Source: CAD feature listing. Evaluate the final solid. Frame: model axes, mm. A direction names the side the tool comes from. Coordinates: 2 decimals unless noted, no trailing zeros. Loops run counter-clockwise (first coordinate to the right, second up) from the corner with the lowest first, then second, coordinate; pieces in that order, holes last.
Item 1: Section query C-C, the plane x = 50. Return the cut outline in (y, z), then the cut area to 3 significant figures.
Item 2: Pull-direction query (Y, two-part tool) for faces 3 (the cylindrical face through (8.73, 42.03, 1.52)), 4 (the flat face through (30, 53, 1)), 5 (the flat face through (0, 26, 1)), 6 (the cylindrical face through (59, 2, 2)); classes: +Y half, -Y half, draft (parallel to the pull), parting line (faces both ways), or undercut.
Item 3: Reachability of faces 1 (the flat face through (60, 26, 1)), 2 (the flat face through (40, 24, 2)) from +Z, -Z, +X, -X, +Y, -Y: full face, straight path, thin tool, end or side. Return the list, or none.
Item 4: Section query D-D, the plane z = 0.65. Return the cut outline in (x, y).
Item 5: Section query B-B, the plane y = 32.5. Return the cut outline in (x, z).
Item 6: Line query: probe 1 along Y at (x, z) = (10, 1.2); probe 2 along Y at (x, z) = (50, 1.9); probe 3 along X at (y, z) = (20.5, 0.15). Output: solid intervals per line, ascending.
Item 7: Section query A-A, the plane x = 10. Return the cut outline in (y, z), then the cut area to 3 significant figures.
Item 8: Pin query (flat end, axial travel): pin 1 Ø2.5 at (x, y) = (50, 30) entering from -Z; pin 2 Ø0.9 at (x, z) = (30, 2) entering from -Y. Return the tip coordinate at first contact, or that it passes through.
```python
from build123d import *

# Parameters (mm, degrees)
SKETCH_1_W          = 60
SKETCH_1_H          = 53
EXTRUDE_1_DEPTH     = 3
SKETCH_2_W          = 20
SKETCH_2_H          = 43
CUT_EXTRUDE_1_DEPTH = 81.112421009
SKETCH_3_R          = 1.6
CUT_EXTRUDE_2_DEPTH = 81.112421009
SKETCH_4_R          = 1.6
CUT_EXTRUDE_3_DEPTH = 81.112421009
FILLET_1_R          = 5
SKETCH_5_R          = 1.6
CUT_EXTRUDE_4_DEPTH = 81.112421009


with BuildPart() as part:
    # 草图1 → 凸台-拉伸1 (new body)
    with BuildSketch(Plane.XY):
        with Locations((30, 26.5)):
            Rectangle(SKETCH_1_W, SKETCH_1_H)
    extrude(amount=EXTRUDE_1_DEPTH)

    # 草图2 → 切除-拉伸1 (cut, through all)
    with BuildSketch(Plane.XY.offset(3)):
        with Locations((30, 21.5)):
            Rectangle(SKETCH_2_W, SKETCH_2_H)
    extrude(amount=-CUT_EXTRUDE_1_DEPTH, mode=Mode.SUBTRACT)

    # 草图3 → 切除-拉伸2 (cut, through all)
    with BuildSketch(Plane.XY.offset(3)):
        with Locations((50, 10)):
            Circle(SKETCH_3_R)
        with Locations((50, 30)):
            Circle(SKETCH_3_R)
        with Locations((50, 48)):
            Circle(SKETCH_3_R)
    extrude(amount=-CUT_EXTRUDE_2_DEPTH, mode=Mode.SUBTRACT)

    # 草图4 → 切除-拉伸3 (cut, through all)
    with BuildSketch(Plane.XY.offset(3)):
        with Locations((10, 10)):
            Circle(SKETCH_4_R)
    extrude(amount=-CUT_EXTRUDE_3_DEPTH, mode=Mode.SUBTRACT)

    # 圆角1
    fillet_1_edges = [part.edges().sort_by_distance(p)[0] for p in [
        (20, 0, 1.5),
        (40, 0, 1.5),
        (0, 53, 1.5),
        (60, 53, 1.5),
        (60, 0, 1.5),
        (0, 0, 1.5),
    ]]
    fillet(fillet_1_edges, radius=FILLET_1_R)

    # 草图5 → 切除-拉伸4 (cut, through all)
    with BuildSketch(Plane.XY.offset(3)):
        with Locations((10, 43)):
            Circle(SKETCH_5_R)
    extrude(amount=-CUT_EXTRUDE_4_DEPTH, mode=Mode.SUBTRACT)


solid = part.part
```
Verdict:
1. outline: (0, 0) - (8.4, 0) - (8.4, 3) - (0, 3) - close; (11.6, 0) - (28.4, 0) - (28.4, 3) - (11.6, 3) - close; (31.6, 0) - (46.4, 0) - (46.4, 3) - (31.6, 3) - close; (49.6, 0) - (53, 0) - (53, 3) - (49.6, 3) - close
1. area: 130 mm2
2. face 3: undercut
2. face 4: +Y half
2. face 5: draft
2. face 6: -Y half
3. face 1: +Z, -Z, +X, +Y, -Y
3. face 2: +Z, -Z, -Y
4. outline: (0, 5) arc R5 ccw to (5, 0) - (15, 0) arc R5 ccw to (20, 5) - (20, 43) - (40, 43) - (40, 5) arc R5 ccw to (45, 0) - (55, 0) arc R5 ccw to (60, 5) - (60, 48) arc R5 ccw to (55, 53) - (5, 53) arc R5 ccw to (0, 48) - close; hole circle Ø3.2 at (10, 10); hole circle Ø3.2 at (10, 43); hole circle Ø3.2 at (50, 10); hole circle Ø3.2 at (50, 30); hole circle Ø3.2 at (50, 48)
5. outline: (0, 0) - (20, 0) - (20, 3) - (0, 3) - close; (40, 0) - (60, 0) - (60, 3) - (40, 3) - close
6. probe 1: y = 0 to 8.4, 11.6 to 41.4, 44.6 to 53
6. probe 2: y = 0 to 8.4, 11.6 to 28.4, 31.6 to 46.4, 49.6 to 53
6. probe 3: x = 0 to 20, 40 to 60
7. outline: (0, 0) - (8.4, 0) - (8.4, 3) - (0, 3) - close; (11.6, 0) - (41.4, 0) - (41.4, 3) - (11.6, 3) - close; (44.6, 0) - (53, 0) - (53, 3) - (44.6, 3) - close
7. area: 140 mm2
8. pin 1: passes through
8. pin 2: stops at y = 43
